Input: dimensioned drawing with shaded views. Units: mm. Origin: part minimum x, y, z. Give positions to 0.01 mm unless a question says otherwise; leave off trailing zeros. Write each loop counter-clockwise with the first axis right and the second up, starting at its lowest first coordinate (ties: lowest second). Pieces come first, ordered by that corner, then holes. Notation, with made-up numbers: (63.25, 28.5) -> (89.25, 28.5) arc R25 ccw to (89.25, 56.5) -> close; hole circle Ø3 at (-32, 57.25). An arc over 180 degrees is marked (long way). Return JSON: item names as keys, results as strings. Group by question number.
Item 1: Section D-D, the plane y = 8.8. Return loops of the section in (x, z).
Item 2: Line query: line 1 (Y direction, x = 8.75, z = 1.6); line 2 (X direction, y = 4.5, z = 2.3); line 3 (Y direction, x = 6, z = 1.05). Output: solid intervals per line, ascending. Write a range as [from, to].
Item 3: Mould query, pull axis X, two halves, no side actions, for the marked faces 1, 2 and 3. Classes: released by +X, released by -X, zero draft, split by the parting line, or undercut.
Item 4: Section A-A, the plane y = 6. Return loops of the section in (x, z), then the cut area to 4 significant figures.
Item 5: Section C-C, the plane z = 4.1. Return loops of the section in (x, y).
Item 6: Pin query (flat end, axial travel): P1, Ø1, axis at y = 5.5, z = 1.5, coming from the +X side; P2, Ø1.5, axis at x = 10, z = 0.5, coming from the -Y side; P3, Ø1.5, axis at x = 3, z = 3, coming from the -Y side; P4, Ø2, axis at y = 1.5, z = 2.5, coming from the -X side. Return the tip coordinate at first contact, or that it passes through.
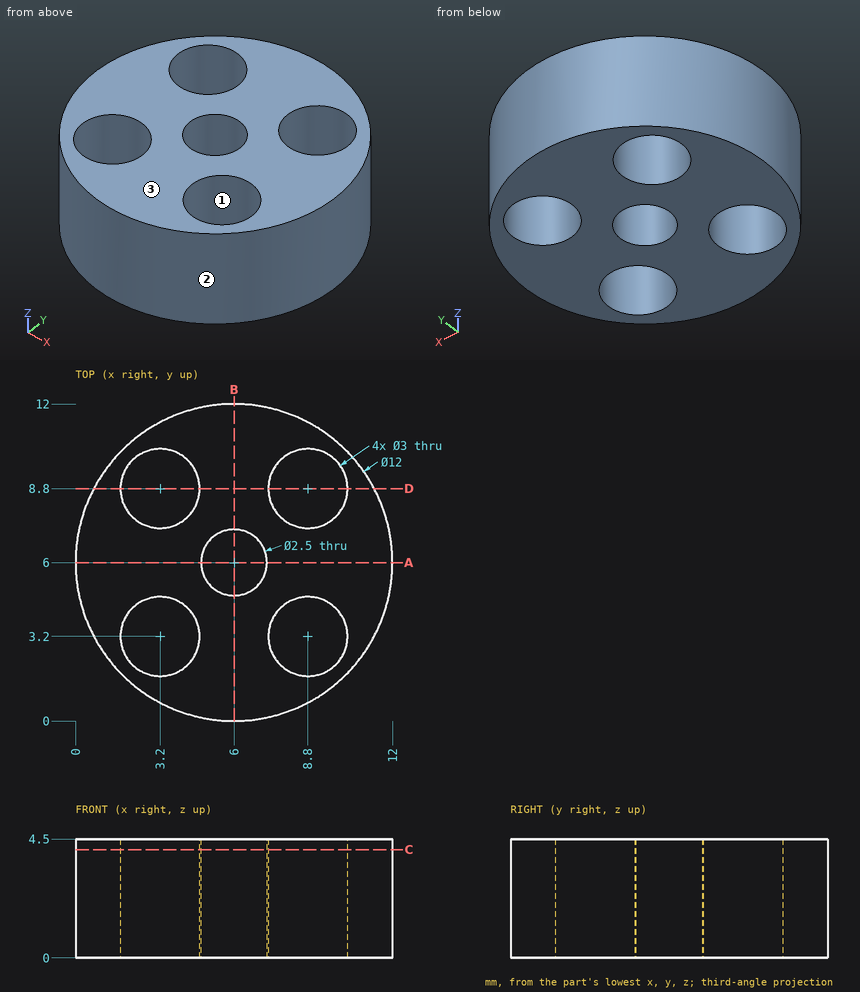
Answer below:
{
 "1": {"outline": "(0.69, 0) -> (1.7, 0) -> (1.7, 4.5) -> (0.69, 4.5) -> close; (4.7, 0) -> (7.3, 0) -> (7.3, 4.5) -> (4.7, 4.5) -> close; (10.3, 0) -> (11.31, 0) -> (11.31, 4.5) -> (10.3, 4.5) -> close"},
 "2": {"line 1": "y = [0.67, 1.7], [4.7, 7.3], [10.3, 11.33]", "line 2": "x = [0.19, 2.45], [3.95, 8.05], [9.55, 11.81]", "line 3": "y = [0, 4.75], [7.25, 12]"},
 "3": {"face 1": "undercut", "face 2": "split by the parting line", "face 3": "zero draft"},
 "4": {"outline": "(0, 0) -> (4.75, 0) -> (4.75, 4.5) -> (0, 4.5) -> close; (7.25, 0) -> (12, 0) -> (12, 4.5) -> (7.25, 4.5) -> close", "area": "42.75 mm2"},
 "5": {"outline": "circle Ø12 at (6, 6); hole circle Ø3 at (3.2, 3.2); hole circle Ø3 at (3.2, 8.8); hole circle Ø2.5 at (6, 6); hole circle Ø3 at (8.8, 3.2); hole circle Ø3 at (8.8, 8.8)"},
 "6": {"P1": "stops at x = 12", "P2": "stops at y = 0.96", "P3": "stops at y = 0.44", "P4": "stops at x = 1.13"}
}
